from build123d import *

# Parameters (mm, degrees)
SKETCH_1_R          = 4.5
EXTRUDE_1_DEPTH     = 40
SKETCH_2_R          = 6.5
EXTRUDE_2_DEPTH     = 8
CUT_EXTRUDE_1_DEPTH = 4


with BuildPart() as part:
    # 스케치1 → 보스-돌출1 (new body)
    with BuildSketch(Plane.XY):
        Circle(SKETCH_1_R)
    extrude(amount=EXTRUDE_1_DEPTH)

    # 스케치2 → 보스-돌출2 (add)
    with BuildSketch(Plane(origin=(0, 0, 0), x_dir=(-1, 0, 0), z_dir=(0, 0, -1))):
        Circle(SKETCH_2_R)
    extrude(amount=EXTRUDE_2_DEPTH)

    # 스케치3 → 컷-돌출1 (cut)
    with BuildSketch(Plane(origin=(0, 0, -8), x_dir=(-1, 0, 0), z_dir=(0, 0, -1))):
        with BuildLine():
            Line((1.51655612, -2.298562783), (2.733251781, -0.335660595))
            ThreePointArc((2.733251781, -0.335660595), (2.80802632, -0.087878298), (2.748891822, 0.164094734))
            Line((2.748891822, 0.164094734), (1.657316493, 2.19923518))
            ThreePointArc((1.657316493, 2.19923518), (1.480117999, 2.387882979), (1.232335703, 2.462657518))
            Line((1.232335703, 2.462657518), (-1.075935288, 2.534895775))
            ThreePointArc((-1.075935288, 2.534895775), (-1.327908321, 2.475761277), (-1.51655612, 2.298562783))
            Line((-1.51655612, 2.298562783), (-2.733251781, 0.335660595))
            ThreePointArc((-2.733251781, 0.335660595), (-2.80802632, 0.087878298), (-2.748891822, -0.164094734))
            Line((-2.748891822, -0.164094734), (-1.657316493, -2.19923518))
            ThreePointArc((-1.657316493, -2.19923518), (-1.480117999, -2.387882979), (-1.232335703, -2.462657518))
            Line((-1.232335703, -2.462657518), (1.075935288, -2.534895775))
            ThreePointArc((1.075935288, -2.534895775), (1.327908321, -2.475761277), (1.51655612, -2.298562783))
        make_face()
    extrude(amount=-CUT_EXTRUDE_1_DEPTH, mode=Mode.SUBTRACT)


solid = part.part
Design review of the part built by this model. Coordinates are the model's own, in mm. A direction names the side the tool comes from. Give positions to 0.01 mm unless a question says otherwise; leave off trailing zeros. Write each loop counter-clockwise with the first axis right and the second up, starting at its lowest first coordinate (ties: lowest second). Pieces come first, ordered by that corner, then holes. Notation, with made-up numbers: M 83.5,62.25 L 115.5,62.25 A18 ccw 115.5,96.25 Z; hole C -22.5,5 d8. An arc over 180 degrees is marked long. Answer as a JSON object with one key per item and string values. Group by question number.
1) We need section C-C (z = -2). Give the boundary of the cut face in (x, y).
2) Tool access review of faces 4 (the face through (-2.21, 1.17, -6.03)), 5 (the face through (-3, 0, -8)): name each direction out of +Z, -Z, +X, -X, +Y, -Y from which nothing blocks a thin tool from reaching the whole face with its end or side.
3) Clearance check with flat-ended pins moving along their axes: pin 1 Ø2 at (y, z) = (-2, 19) entering from +X; pin 2 Ø3 at (x, z) = (-2.5, 34) entering from -Y; pin 3 Ø5 at (y, z) = (3, 33) entering from -X. State where each tip first meets the part, or that it passes through.
4) We need section A-A (x = -0.5). Give the boundary of the cut face in (y, z), and give its area (3 significant figures).
5) We need section D-D (x = -4). Give the boundary of the cut face in (y, z), and give its area (3 significant figures).
6) For line 1 along Y through (x, z) = (0.25, 4); line 2 along Z through (x, y) = (1.5, 1.5); line 3 along Z through (x, y) = (5.75, -1.25), list the stretches that pass through material, from the lowest coordinate up.
7) We need section B-B (y = -1.75). Give the boundary of the cut face in (x, z).
8) Mouldability with a two-part tool opening along Y and no side actions: class faces 1 (the face through (4.42, 1.54, 0)), 2 (the face through (-2.116, -1.331, -6.028)), 3 (the face through (-0.59, 4.46, 19.72)) as released by +Y, released by -Y, zero draft, split by the parting line, or undercut.
Answer key:
{
 "1": {"outline": "C 0,0 d13"},
 "2": {"face 4": "-Z", "face 5": "-Z, +X, -X, +Y, -Y"},
 "3": {"pin 1": "stops at x = 4.39", "pin 2": "stops at y = -4.39", "pin 3": "stops at x = -4.47"},
 "4": {"outline": "M -6.48,-8 L -2.52,-8 L -2.52,-4 L 2.49,-4 L 2.49,-8 L 6.48,-8 L 6.48,0 L 4.47,0 L 4.47,40 L -4.47,40 L -4.47,0 L -6.48,0 Z", "area": "441 mm²"},
 "5": {"outline": "M -5.12,-8 L 5.12,-8 L 5.12,0 L 2.06,0 L 2.06,40 L -2.06,40 L -2.06,0 L -5.12,0 Z", "area": "247 mm²"},
 "6": {"line 1": "y = -4.49 to 4.49", "line 2": "z = -4 to 40", "line 3": "z = -8 to 0"},
 "7": {"outline": "M -6.26,-8 L -1.86,-8 L -1.86,-4 L 1.9,-4 L 1.9,-8 L 6.26,-8 L 6.26,0 L 4.15,0 L 4.15,40 L -4.15,40 L -4.15,0 L -6.26,0 Z"},
 "8": {"face 1": "zero draft", "face 2": "undercut", "face 3": "split by the parting line"}
}
